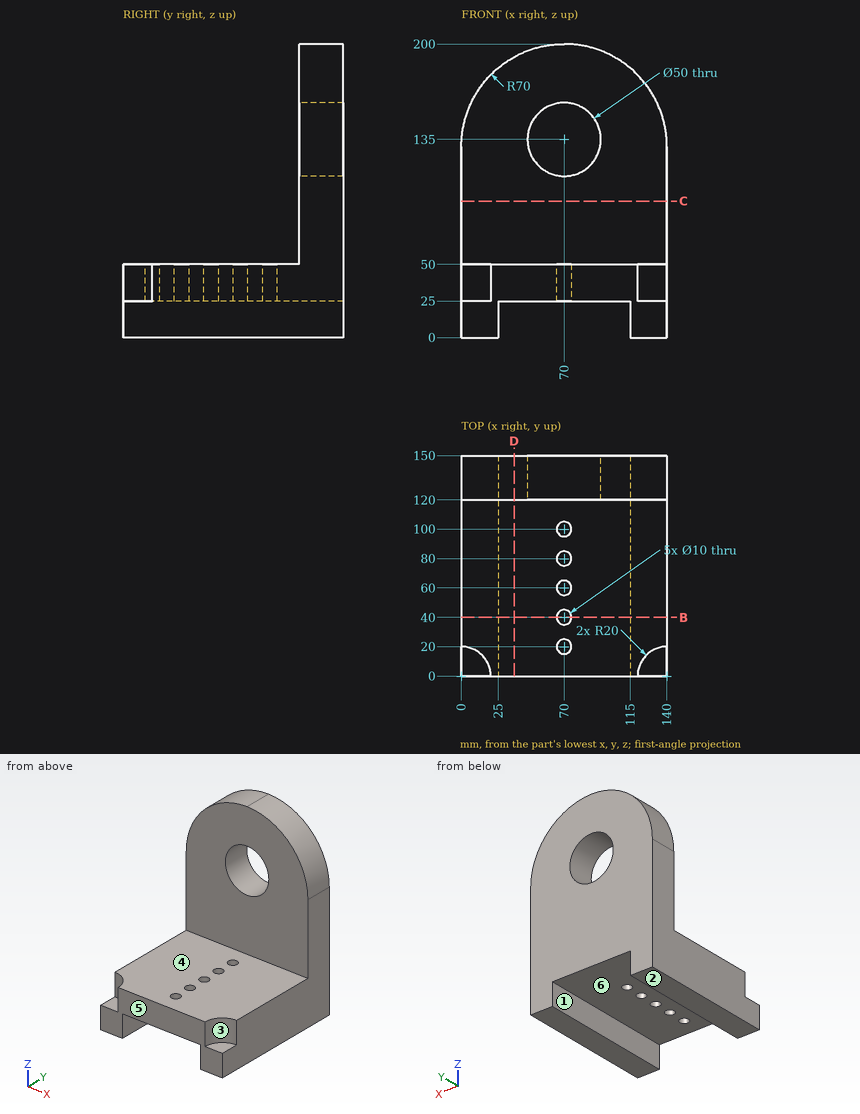
Input: dimensioned drawing with shaded views. Units: mm. Origin: part minimum x, y, z. A direction names the side the tool comes from. Coordinates: 2 decimals unless noted, no trailing zeros. Loops run counter-clockwise (first coordinate to the right, second up) from the corner with the lowest first, then second, coordinate; pieces in that order, holes last. Notation, with made-up numbers: M 26.5,-34.75 L 72.5,-34.75 A26 ccw 72.5,4.25 Z; hole C 47.5,67.25 d11. An arc over 180 degrees is marked long. Use a Markdown table: item, result. Add a question column.
Q1. Material intervals for L1, parallel to Y at x = 70, z = 35.75; L2, parallel to X at y = 58, z = 23.5; L3, parallel to Z at x = 62, y = 35, sorted ascending.
Q2. First-contact query: pin 1 (16 mm diameter, centred on x = 70, y = 40, fed in from +Z); pin 2 (6 mm diameter, centred on x = 112.5, z = 110, fed in from -Y); pin 3 (9 mm diameter, centred on x = 70, y = 100, fed in from +Z); pin 4 (11.5 mm diameter, centred on x = 70, y = 80, fed in from -Z). Flat tips, straight axial feed; report the tip coordinate or a pass-through.
Q3. Draft query along X for the marked faces 1, 2 and 3. Return one class per face: pulls with the +X half, pulls with the -X half, needs draft (parallel to the pull), parting line crosses it, or undercut.
Q4. Section query D-D, the plane x = 36. Return loops of the section in (y, z), and give its area (3 significant figures).
Q5. Section query C-C, the plane z = 93. Return loops of the section in (x, y).
Q6. Section query B-B, the plane y = 40. Return loops of the section in (x, z).
Q7. Access query for the marked faces 4, 5 and 6. Directions: +Z, -Z, +X, -X, +Y, -Y. A direction counts if a zero-diameter tool reaches every point of the face in a straight line with its end or side. Return the directions, or none.
Result:
| question | item | result |
|---|---|---|
| 1 | L1 | y = 0 to 15, 25 to 35, 45 to 55, 65 to 75, 85 to 95, 105 to 150 |
| 1 | L2 | x = 0 to 25, 115 to 140 |
| 1 | L3 | z = 25 to 50 |
| 2 | pin 1 | stops at z = 50 |
| 2 | pin 2 | stops at y = 120 |
| 2 | pin 3 | passes through |
| 2 | pin 4 | stops at z = 25 |
| 3 | face 1 | undercut |
| 3 | face 2 | needs draft |
| 3 | face 3 | pulls with the +X half |
| 4 | outline | M 0,25 L 150,25 L 150,191.19 L 120,191.19 L 120,50 L 0,50 Z |
| 4 | area | 7,990 mm2 |
| 5 | outline | M 0,120 L 140,120 L 140,150 L 0,150 Z |
| 6 | outline | M 0,0 L 25,0 L 25,25 L 65,25 L 65,50 L 0,50 Z; M 75,25 L 115,25 L 115,0 L 140,0 L 140,50 L 75,50 Z |
| 7 | face 4 | +Z, +X, -X, -Y |
| 7 | face 5 | +Z, -Z, +X, -X, -Y |
| 7 | face 6 | -Z, +Y, -Y |
